Input: part model. Units: mm. Frame: model coordinates. Face numbers are marked on the shaded views. Give positions to 0.01 mm unless a question says otherwise; leave off trailing zeros. Loops run counter-clockwise (first coordinate to the right, second up) from the corner with the lowest first, then second, coordinate; pieces in that order, holes last. Notation, with made-up numbers: (35.5, 31.25) - (58.5, 31.25) arc R13 cw to (58.5, 56.25) - close; hole circle Ø1 at (-6, -12.5). An arc over 180 degrees is marked (long way). Answer as a JSON object with one key per item and string values. Group by question number.
(1) Material intervals for L1, parallel to Y at x = 2.75, z = -2.5; L2, parallel to Y at x = 0, z = -12.75; L3, parallel to X at y = 0.75, z = -12.75, sorted ascending.
(2) Section query A-A (z = -13.25). Return loops of the section in (x, y), plus the area to 3 significant figures.
(3) Pin query (flat end, axial travel): P1, Ø2, axis at y = 2.5, z = -6.5, coming from the -X side; P2, Ø2, axis at x = 2.5, z = -7, coming from the -Y side; P3, Ø1, axis at x = -2, z = -13.5, coming from the -Y side. Return the tip coordinate at first contact, or that it passes through.
(4) Mould query, pull axis Y, two halves, no side actions, for the marked faces 1, 2, 3 and 4. Classes: +Y half, -Y half, draft (parallel to the pull), parting line (faces both ways), or undercut.
(5) Section query B-B (z = -9.75). Return loops of the section in (x, y), plus the area to 3 significant figures.
```python
from build123d import *

# Parameters (mm, degrees)
F_6_0MM_DOWEL_HOLE1_D     = 6
F_6_0MM_DOWEL_HOLE1_DEPTH = 9
F_6_0MM_DOWEL_HOLE1_TIP   = 1.802581857
CUT_EXTRUDE1_DEPTH        = 10
CUT_EXTRUDE1_DEPTH_BACK   = 10
SKETCH4_R                 = 1


with BuildPart() as part:
    # Sketch1 → Revolve1 (revolve)
    with BuildSketch(Plane(origin=(0, 0, 0), x_dir=(1, 0, 0), z_dir=(0, 1, 0)), mode=Mode.PRIVATE) as revolve1_sk:
        with BuildLine():
            Line((0, 0), (-0.766214157, 0))
            ThreePointArc((-0.766214157, 0), (-4.301748063, 1.464466094), (-5.766214157, 5))
            Line((-5.766214157, 5), (-5.766214157, 6))
            Line((-5.766214157, 6), (-6.75, 13))
            Line((-6.75, 13), (-6.75, 15))
            Line((-6.75, 15), (0, 15))
            Line((0, 15), (0, 0))
        make_face()
    revolve(revolve1_sk.sketch.rotate(Axis((0, 0, 0), (0, 0, -1)), 180), axis=Axis((0, 0, 0), (0, 0, -1)))

    # 6.0mm Dowel Hole1
    with Locations(Plane(origin=(0, 0, -15), x_dir=(-1, 0, 0), z_dir=(0, 0, -1))):
        with Locations((0, 0)):
            Hole(F_6_0MM_DOWEL_HOLE1_D / 2, depth=F_6_0MM_DOWEL_HOLE1_DEPTH)
            with Locations((0, 0, -(F_6_0MM_DOWEL_HOLE1_DEPTH + F_6_0MM_DOWEL_HOLE1_TIP / 2))):  # 118° drill point
                Cone(0, F_6_0MM_DOWEL_HOLE1_D / 2, F_6_0MM_DOWEL_HOLE1_TIP, mode=Mode.SUBTRACT)

    # Sketch4 → Cut-Extrude1 (cut, two sides: drawn at the far end of the back side and taken through both)
    with BuildSketch(Plane(origin=(0, 0, 0), x_dir=(0, 0, -1), z_dir=(1, 0, 0)).offset(-CUT_EXTRUDE1_DEPTH_BACK)):
        with Locations(Location((2.103245374, 0, 0), (0, 0, 179.99999994))):
            Circle(SKETCH4_R)
    extrude(amount=CUT_EXTRUDE1_DEPTH + CUT_EXTRUDE1_DEPTH_BACK, mode=Mode.SUBTRACT)


solid = part.part
```
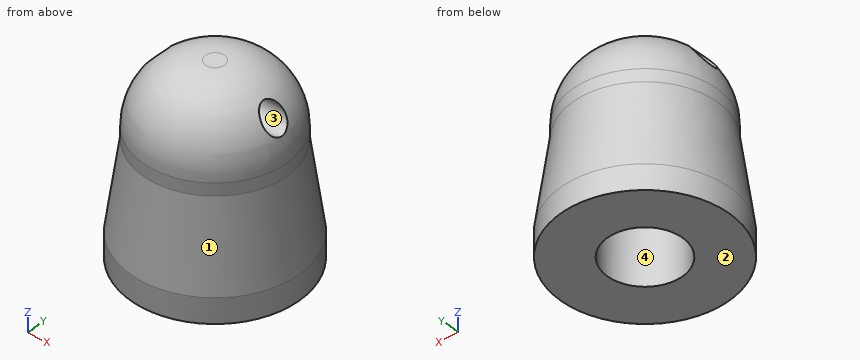
Recorded:
{
 "1": {"L1": "y = -4.29 to -0.92, 0.92 to 4.29", "L2": "y = -6.71 to -3, 3 to 6.71", "L3": "x = -6.67 to -2.9, 2.9 to 6.67"},
 "2": {"outline": "circle Ø13.5 at (0, 0); hole circle Ø6 at (0, 0)", "area": "115 mm^2"},
 "3": {"P1": "stops at x = -5.68", "P2": "stops at y = -5.75", "P3": "stops at y = -6.58"},
 "4": {"face 1": "parting line", "face 2": "draft", "face 3": "undercut", "face 4": "undercut"},
 "5": {"outline": "circle Ø12.59 at (0, 0); hole circle Ø6 at (0, 0)", "area": "96.1 mm^2"}
}
